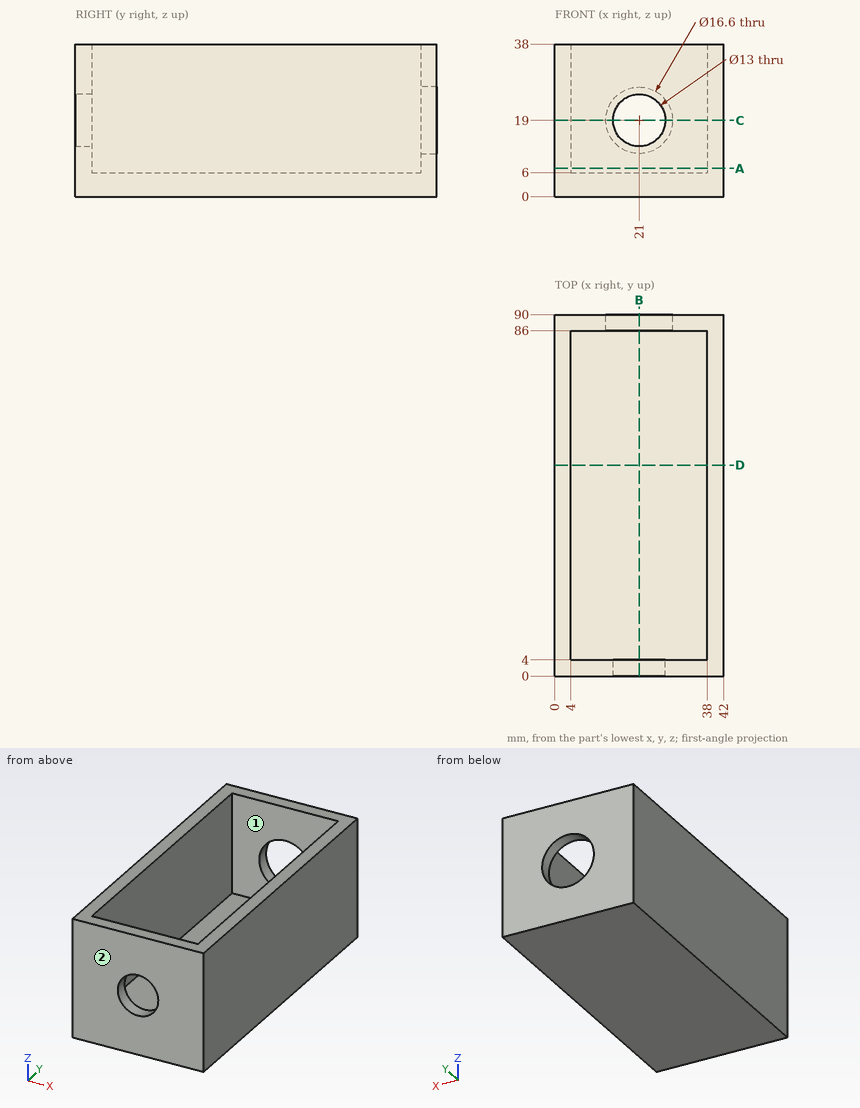
Geometry: see drawing. Coordinates: mm, zero at the bounding-box minimum. A direction names the side the tool comes from. Give positions to 0.01 mm unless a question says otherwise; leave off trailing zeros. Loops run counter-clockwise (first coordinate to the right, second up) from the corner with the lowest first, then second, coordinate; pieces in that order, holes last. Notation, with made-up numbers: (16.25, 52) -> (24.25, 52) arc R7 cw to (24.25, 61) -> close; hole circle Ø1 at (64, 44). An arc over 180 degrees is marked (long way). Put each result on its own line as item: value.
1. Cut plane D-D (y = 52.5). Return the cut outline in (x, z), plus the area to 3 significant figures.
Taken from the geometry:
outline: (0, 0) -> (42, 0) -> (42, 38) -> (38, 38) -> (38, 6) -> (4, 6) -> (4, 38) -> (0, 38) -> close
area: 508 mm2
2. Cut plane B-B (x = 21). Return the cut outline in (y, z), plus the area to 3 significant figures.
Taken from the geometry:
outline: (0, 0) -> (90, 0) -> (90, 10.7) -> (86, 10.7) -> (86, 6) -> (4, 6) -> (4, 12.5) -> (0, 12.5) -> close; (0, 25.5) -> (4, 25.5) -> (4, 38) -> (0, 38) -> close; (86, 27.3) -> (90, 27.3) -> (90, 38) -> (86, 38) -> close
area: 678 mm2
3. Set-up query: the marked faces 1 and 2. Return all of +Z, -Z, +X, -X, +Y, -Y with unobstructed straight access to the full face (end or side cutting, diameter ignored); none if empty.
Taken from the geometry:
face 1: +Z
face 2: +Z, -Z, +X, -X, -Y
4. Cut plane C-C (z = 19). Return the cut outline in (x, y).
Taken from the geometry:
outline: (0, 0) -> (14.5, 0) -> (14.5, 4) -> (4, 4) -> (4, 86) -> (12.7, 86) -> (12.7, 90) -> (0, 90) -> close; (27.5, 0) -> (42, 0) -> (42, 90) -> (29.3, 90) -> (29.3, 86) -> (38, 86) -> (38, 4) -> (27.5, 4) -> close
5. Cut plane A-A (z = 7). Return the cut outline in (x, y).
Taken from the geometry:
outline: (0, 0) -> (42, 0) -> (42, 90) -> (0, 90) -> close; hole (4, 4) -> (38, 4) -> (38, 86) -> (4, 86) -> close
6. Ray query, line 1 along Y through (x, z) = (21, 29.5); line 2 along X through (y, z) = (19, 22); line 3 along X through (y, z) = (88, 19). Return the intervals inside material, ascending. Write a range as [from, to].
Taken from the geometry:
line 1: y = [0, 4], [86, 90]
line 2: x = [0, 4], [38, 42]
line 3: x = [0, 12.7], [29.3, 42]
7. Pin query (flat end, axial travel): P1, Ø11.5, axis at x = 21, z = 19, coming from the +Y side. Return the tip coordinate at first contact, or that it passes through.
Taken from the geometry:
P1: passes through
